Could you check a few things on this drawing? It's one solid part, dimensions in mm from its lowest x, y, z. A direction names the side the tool comes from. Give positions to 0.01 mm unless a question says otherwise; leave off trailing zeros. Loops run counter-clockwise (first coordinate to the right, second up) from the corner with the lowest first, then second, coordinate; pieces in that order, holes last. Notation, with made-up numbers: M 47,-20.5 L 88,-20.5 A20 cw 88,9.5 Z; hole C 53.5,-34 d9. An arc over 180 degrees is marked long. Answer in a Markdown table with one row per item. Add a question column.
1. If we section it at C-C on z = 11: List the corners of the cut face in (x, y) for me, then the cut area to 3 significant figures.
2. I'm going to push flat-ended pins straight in: pin 1 Ø5 at (x, y) = (6.5, 54) entering from +Z; pin 2 Ø1.3 at (x, y) = (68.5, 18) entering from -Z; pin 3 Ø8 at (x, z) = (18.5, 19) entering from -Y; pin 4 Ø6 at (x, y) = (36, 40) entering from +Z. Where does each tip first touch, or does it pass through?
3. Thinking about a two-plate mould opening in X: for the marked faces 1, 2, 3 and 4, which applies, released by +X, released by -X, zero draft, split by the parting line, or undercut?
4. I need wall thicknesses on line 1 along Y through (x, z) = (68.5, 1.7); line 2 along X through (y, z) = (18, 2.1); line 3 along X through (y, z) = (5, 12.5). Which ranges of each line are inside material? Lowest first, please. Write a range as from..to.
5. Which directions (+Z, -Z, +X, -X, +Y, -Y) give clear straight access to the entire face, cutting with the end or side of a thin tool? Please do the marked faces 5 and 6.
6. If we section it at A-A on x = 6.5: List the corners of the cut face in (y, z) for me.
7. If we section it at D-D on x = 42: List the corners of the cut face in (y, z) for me, then the cut area to 3 significant figures.
8. If we section it at B-B on y = 54: List the corners of the cut face in (x, z) for me.
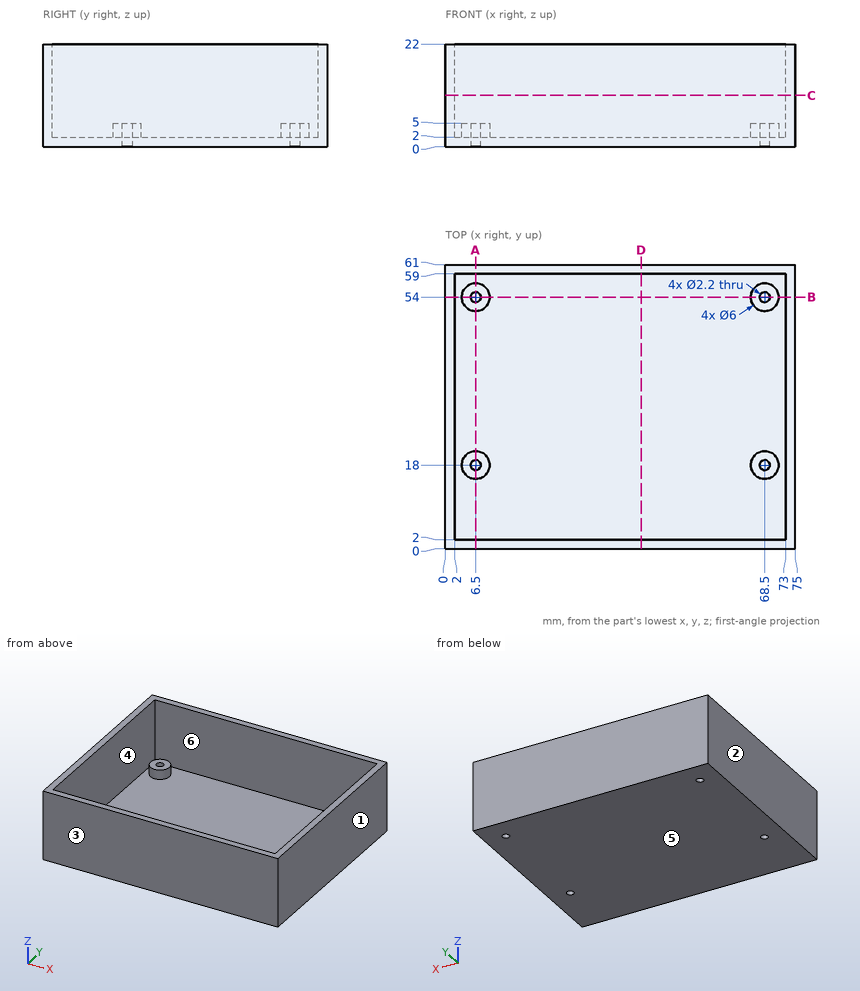
Results:
| question | item | result |
|---|---|---|
| 1 | outline | M 0,0 L 75,0 L 75,61 L 0,61 Z; hole M 2,2 L 73,2 L 73,59 L 2,59 Z |
| 1 | area | 528 mm2 |
| 2 | pin 1 | z = 5 |
| 2 | pin 2 | through |
| 2 | pin 3 | y = 0 |
| 2 | pin 4 | z = 2 |
| 3 | face 1 | released by +X |
| 3 | face 2 | released by -X |
| 3 | face 3 | zero draft |
| 3 | face 4 | undercut |
| 4 | line 1 | 0..16.9, 19.1..52.9, 55.1..61 |
| 4 | line 2 | 0..2, 3.5..5.4, 7.6..9.5, 65.5..67.4, 69.6..71.5, 73..75 |
| 4 | line 3 | 0..2, 73..75 |
| 5 | face 5 | -Z, +X, -X, +Y, -Y |
| 5 | face 6 | +Z |
| 6 | outline | M 0,0 L 16.9,0 L 16.9,5 L 15,5 L 15,2 L 2,2 L 2,22 L 0,22 Z; M 19.1,0 L 52.9,0 L 52.9,5 L 51,5 L 51,2 L 21,2 L 21,5 L 19.1,5 Z; M 55.1,0 L 61,0 L 61,22 L 59,22 L 59,2 L 57,2 L 57,5 L 55.1,5 Z |
| 7 | outline | M 0,0 L 61,0 L 61,22 L 59,22 L 59,2 L 2,2 L 2,22 L 0,22 Z |
| 7 | area | 202 mm2 |
| 8 | outline | M 0,0 L 5.4,0 L 5.4,5 L 3.5,5 L 3.5,2 L 2,2 L 2,22 L 0,22 Z; M 7.6,0 L 67.4,0 L 67.4,5 L 65.5,5 L 65.5,2 L 9.5,2 L 9.5,5 L 7.6,5 Z; M 69.6,0 L 75,0 L 75,22 L 73,22 L 73,2 L 71.5,2 L 71.5,5 L 69.6,5 Z |
